```python
from build123d import *

# Parameters (mm, degrees)
BOSS_EXTRUDE4_DEPTH = 6
BOSS_EXTRUDE6_DEPTH = 12
BOSS_EXTRUDE7_START = 12
SKETCH7_R           = 11
BOSS_EXTRUDE7_DEPTH = 12


with BuildPart() as part:
    # Sketch2 → Boss-Extrude4 (new body)
    with BuildSketch(Plane.XY):
        with BuildLine():
            Line((-50, 22), (50, 22))
            ThreePointArc((50, 22), (72, 0), (50, -22))
            Line((50, -22), (-50, -22))
            ThreePointArc((-50, -22), (-72, 0), (-50, 22))
        make_face()
    extrude(amount=BOSS_EXTRUDE4_DEPTH)

    # Sketch5 → Boss-Extrude6 (add)
    with BuildSketch(Plane.XY.offset(6)):
        with BuildLine():
            Line((-40.780455543, 6), (71.166010489, 6))
            ThreePointArc((71.166010489, 6), (72, 0), (71.166010489, -6))
            Line((71.166010489, -6), (-40.780455543, -6))
            ThreePointArc((-40.780455543, -6), (-39, 0), (-40.780455543, 6))
        make_face()
    extrude(amount=BOSS_EXTRUDE6_DEPTH)

    # Sketch7 → Boss-Extrude7 (add)
    with BuildSketch(Plane(origin=(0, 0, 0), x_dir=(-1, 0, 0), z_dir=(0, 0, -1)).offset(BOSS_EXTRUDE7_START)):
        with Locations(Location((50, 0, 0), (0, 0, 180))):
            Circle(SKETCH7_R)
    extrude(amount=-BOSS_EXTRUDE7_DEPTH)


solid = part.part
```
Geometry check sheet. Reference: the model listing, model coordinates, mm. A direction names the side the tool comes from. Give positions to 0.01 mm unless a question says otherwise; leave off trailing zeros. Order: outer loops, then holes, each group sorted by start corner. A loop starts at its lowest first (then second) coordinate and runs counter-clockwise, first axis right, second up.
1. Access from +Z, -Z, +X, -X, +Y, -Y to the whole of each face (thin tool, end or side, straight path). Record for faces 1 (the face through (14, 6, 12)), 2 (the face through (16, -6, 12)), 3 (the face through (1, -22, 3)).
2. Section check A-A, the plane x = 5. Enter the section's corners in (y, z).
3. Section check C-C, the plane z = 8.75. Enter the section's corners in (x, y), and give its area (3 significant figures).
4. Release check for a two-part mould opening along Y. For faces 4 (the face through (-39.839, 4.213, -6.084)), 5 (the face through (-39, 0, 12)), 6 (the face through (1, 0, 0)) record: pulls with the +Y half, pulls with the -Y half, needs draft (parallel to the pull), parting line crosses it, or undercut.
5. Gauge pin test, flat ends, axial feed: pin 1 Ø6 at (y, z) = (0, 10) entering from -X; pin 2 Ø1.5 at (y, z) = (1.5, 15) entering from -X; pin 3 Ø2 at (y, z) = (15.5, 2.5) entering from +X. Record the tip position at first contact, or that the pin passes through.
6. Section check D-D, the plane x = -59. Enter the section's corners in (y, z), and give its area (3 significant figures).
7. Section check B-B, the plane y = 0. Enter the section's corners in (x, z).
8. Thickness scan on L1, parallel to Z at x = 4.5, y = 8.5; L2, parallel to Y at x = 50, z = 11; L3, parallel to Z at x = -42.5, y = 3. Record the ranges inside material, lowest first.
Values follow:
1. face 1: +Z, +X, -X, +Y
1. face 2: +Z, +X, -X, -Y
1. face 3: +Z, -Z, +X, -X, -Y
2. outline: (-22, 0) - (22, 0) - (22, 6) - (6, 6) - (6, 18) - (-6, 18) - (-6, 6) - (-22, 6) - close
3. outline: (-40.78, -6) - (71.17, -6) arc R22 ccw to (71.17, 6) - (-40.78, 6) arc R11 cw to start
3. area: 1,340 mm2
4. face 4: parting line crosses it
4. face 5: undercut
4. face 6: needs draft
5. pin 1: stops at x = -39.42
5. pin 2: stops at x = -39.23
5. pin 3: stops at x = 66.55
6. outline: (-20.07, 0) - (-6.32, 0) - (-6.32, -12) - (6.32, -12) - (6.32, 0) - (20.07, 0) - (20.07, 6) - (-20.07, 6) - close
6. area: 393 mm2
7. outline: (-72, 0) - (-61, 0) - (-61, -12) - (-39, -12) - (-39, 0) - (72, 0) - (72, 18) - (-39, 18) - (-39, 6) - (-72, 6) - close
8. L1: z = 0 to 6
8. L2: y = -6 to 6
8. L3: z = -12 to 6
